from build123d import *

# Parameters (mm, degrees)
SKETCH_1_R          = 14
SKETCH_1_R_2        = 1.151350939
EXTRUDE_1_DEPTH     = 4
SKETCH_2_R          = 5.75
EXTRUDE_2_DEPTH     = 12
SKETCH_3_R          = 4
CUT_EXTRUDE_1_DEPTH = 16


with BuildPart() as part:
    # ｽｹｯﾁ1 → ﾎﾞｽ - 押し出し1 (new body)
    with BuildSketch(Plane(origin=(0, 0, 0), x_dir=(0, 0, -1), z_dir=(1, 0, 0))):
        Circle(SKETCH_1_R)
        with Locations((0, 10.5)):
            Circle(SKETCH_1_R_2, mode=Mode.SUBTRACT)
        with Locations((9.09326674, -5.25)):
            Circle(SKETCH_1_R_2, mode=Mode.SUBTRACT)
        with Locations((-9.09326674, -5.25)):
            Circle(SKETCH_1_R_2, mode=Mode.SUBTRACT)
    extrude(amount=EXTRUDE_1_DEPTH)

    # ｽｹｯﾁ2 → ﾎﾞｽ - 押し出し2 (add)
    with BuildSketch(Plane(origin=(4, 0, 0), x_dir=(0, 0, -1), z_dir=(1, 0, 0))):
        Circle(SKETCH_2_R)
    extrude(amount=EXTRUDE_2_DEPTH)

    # ｽｹｯﾁ3 → ｶｯﾄ - 押し出し1 (cut)
    with BuildSketch(Plane(origin=(16, 0, 0), x_dir=(0, 0, -1), z_dir=(1, 0, 0))):
        Circle(SKETCH_3_R)
    extrude(amount=-CUT_EXTRUDE_1_DEPTH, mode=Mode.SUBTRACT)


solid = part.part
Check sheet for the modelled part. Datum: model origin and axes. Units: mm. Give positions to 0.01 mm unless a question says otherwise; leave off trailing zeros. Loops run counter-clockwise (first coordinate to the right, second up) from the corner with the lowest first, then second, coordinate; pieces in that order, holes last. Notation, with made-up numbers: M 47,15 L 91,15 A31 cw 91,44 Z; hole C -29,87 d9. An arc over 180 degrees is marked long. Answer as a JSON object with one key per item and string values. Group by question number.
Q1. Cross-section at A-A on y = 0. Record the cut outline in (x, z), then the cut area to 3 significant figures.
Q2. Material ranges on line 1 along Y through (x, z) = (3.1, 0); line 2 along X through (y, z) = (0.75, -10); line 3 along Y through (x, z) = (7.75, 0), recorded low to high. Write a range as [from, to].
Q3. Cross-section at C-C on x = 13.5. Record the cut outline in (y, z).
Q4. Cross-section at D-D on y = -5.25. Record the cut outline in (x, z), then the cut area to 3 significant figures.
Q5. Release check for a two-part mould opening along Y. For faces 1 (the cylindrical face through (1.97, 11.64, 0.15)), 2 (the cylindrical face through (9.92, 5.7, 0.75)), 3 (the flat face through (4, 0, -6)) record: released by +Y, released by -Y, zero draft, split by the parting line, or undercut.
Q6. Go/stop test with flat-tipped pins: P1, Ø7, axis at y = 0, z = 0, coming from the -X side; P2, Ø5, axis at y = -11, z = -3, coming from the +X side; P3, Ø1.5, axis at x = 5.5, y = -3, coming from the -Z side; P4, Ø1.5, axis at x = 4, z = -10, coming from the +Y side. Record where each tip stops, or that it passes through.
Q7. Cross-section at B-B on z = 0. Record the cut outline in (x, y), then the cut area to 3 significant figures.
Evaluation:
{
 "1": {"outline": "M 0,-14 L 4,-14 L 4,-5.75 L 16,-5.75 L 16,-4 L 0,-4 Z; M 0,4 L 16,4 L 16,5.75 L 4,5.75 L 4,14 L 0,14 Z", "area": "122 mm2"},
 "2": {"line 1": "y = [-14, -4], [4, 9.35], [11.65, 14]", "line 2": "x = [0, 4]", "line 3": "y = [-5.75, -4], [4, 5.75]"},
 "3": {"outline": "C 0,0 d11.5; hole C 0,0 d8"},
 "4": {"outline": "M 0,-12.98 L 4,-12.98 L 4,-10.24 L 0,-10.24 Z; M 0,-7.94 L 4,-7.94 L 4,-2.35 L 16,-2.35 L 16,2.35 L 4,2.35 L 4,7.94 L 0,7.94 Z; M 0,10.24 L 4,10.24 L 4,12.98 L 0,12.98 Z", "area": "142 mm2"},
 "5": {"face 1": "undercut", "face 2": "split by the parting line", "face 3": "zero draft"},
 "6": {"P1": "passes through", "P2": "stops at x = 4", "P3": "stops at z = -5.29", "P4": "stops at y = 10.51"},
 "7": {"outline": "M 0,-14 L 4,-14 L 4,-5.75 L 16,-5.75 L 16,-4 L 0,-4 Z; M 0,4 L 16,4 L 16,5.75 L 4,5.75 L 4,9.35 L 0,9.35 Z; M 0,11.65 L 4,11.65 L 4,14 L 0,14 Z", "area": "113 mm2"}
}
